Work out the finished part from the listing and answer in its coordinate system (mm). Coordinates: 2 decimals unless noted, no trailing zeros. Loops run counter-clockwise (first coordinate to the right, second up) from the corner with the lowest first, then second, coordinate; pieces in that order, holes last. Notation, with made-up numbers: (38.5, 25.5) -> (44.5, 25.5) arc R17 cw to (44.5, 41.5) -> close; hole circle Ø6 at (32.5, 43). An arc over 180 degrees is marked (long way). Use a Markdown table: item, result.
from build123d import *

# Parameters (mm, degrees)
CROQUIS1_W              = 250
CROQUIS1_H              = 150
SALIENTE_EXTRUIR1_DEPTH = 10
CORTAR_EXTRUIR1_REACH   = 12
CROQUIS2_R              = 12.5
CROQUIS2_R_2            = 15.5
CORTAR_EXTRUIR2_REACH   = 12
CROQUIS3_R              = 1.6


with BuildPart() as part:
    # Croquis1 → Saliente-Extruir1 (new body)
    with BuildSketch(Plane(origin=(0, 0, 0), x_dir=(1, 0, 0), z_dir=(0, 1, 0))):
        Rectangle(CROQUIS1_W, CROQUIS1_H)
    extrude(amount=SALIENTE_EXTRUIR1_DEPTH)

    # Croquis2 → Cortar-Extruir1 (cut, up to next)
    with BuildSketch(Plane(origin=(0, 10, 0), x_dir=(1, 0, 0), z_dir=(0, 1, 0)), mode=Mode.PRIVATE) as cortar_extruir1_sk1:
        with Locations((-73.102687588, -7.952940163)):
            Circle(CROQUIS2_R)
    cortar_extruir1_tool1 = extrude(cortar_extruir1_sk1.sketch, amount=-CORTAR_EXTRUIR1_REACH, mode=Mode.PRIVATE) & part.part
    add(cortar_extruir1_tool1.solids().sort_by_distance((-73.102688, 10, 7.95294))[0], mode=Mode.SUBTRACT)
    # Croquis2 → Cortar-Extruir1 (cut, up to next)
    with BuildSketch(Plane(origin=(0, 10, 0), x_dir=(1, 0, 0), z_dir=(0, 1, 0)), mode=Mode.PRIVATE) as cortar_extruir1_sk2:
        with Locations((-4.370803181, -26.878296525)):
            Circle(CROQUIS2_R_2)
    cortar_extruir1_tool2 = extrude(cortar_extruir1_sk2.sketch, amount=-CORTAR_EXTRUIR1_REACH, mode=Mode.PRIVATE) & part.part
    add(cortar_extruir1_tool2.solids().sort_by_distance((-4.370803, 10, 26.878297))[0], mode=Mode.SUBTRACT)
    # Croquis2 → Cortar-Extruir1 (cut, up to next)
    with BuildSketch(Plane(origin=(0, 10, 0), x_dir=(1, 0, 0), z_dir=(0, 1, 0)), mode=Mode.PRIVATE) as cortar_extruir1_sk3:
        with Locations((2.765040009, 12.93083036)):
            Circle(CROQUIS2_R_2)
    cortar_extruir1_tool3 = extrude(cortar_extruir1_sk3.sketch, amount=-CORTAR_EXTRUIR1_REACH, mode=Mode.PRIVATE) & part.part
    add(cortar_extruir1_tool3.solids().sort_by_distance((2.76504, 10, -12.93083))[0], mode=Mode.SUBTRACT)
    # Croquis2 → Cortar-Extruir1 (cut, up to next)
    with BuildSketch(Plane(origin=(0, 10, 0), x_dir=(1, 0, 0), z_dir=(0, 1, 0)), mode=Mode.PRIVATE) as cortar_extruir1_sk4:
        with Locations((39.781486463, 27.243051559)):
            Circle(CROQUIS2_R_2)
    cortar_extruir1_tool4 = extrude(cortar_extruir1_sk4.sketch, amount=-CORTAR_EXTRUIR1_REACH, mode=Mode.PRIVATE) & part.part
    add(cortar_extruir1_tool4.solids().sort_by_distance((39.781486, 10, -27.243052))[0], mode=Mode.SUBTRACT)
    # Croquis2 → Cortar-Extruir1 (cut, up to next)
    with BuildSketch(Plane(origin=(0, 10, 0), x_dir=(1, 0, 0), z_dir=(0, 1, 0)), mode=Mode.PRIVATE) as cortar_extruir1_sk5:
        with Locations((76.517860202, 27.243051559)):
            Circle(CROQUIS2_R_2)
    cortar_extruir1_tool5 = extrude(cortar_extruir1_sk5.sketch, amount=-CORTAR_EXTRUIR1_REACH, mode=Mode.PRIVATE) & part.part
    add(cortar_extruir1_tool5.solids().sort_by_distance((76.51786, 10, -27.243052))[0], mode=Mode.SUBTRACT)
    # Croquis2 → Cortar-Extruir1 (cut, up to next)
    with BuildSketch(Plane(origin=(0, 10, 0), x_dir=(1, 0, 0), z_dir=(0, 1, 0)), mode=Mode.PRIVATE) as cortar_extruir1_sk6:
        with Locations((68.851282971, -12.913044543)):
            Circle(CROQUIS2_R_2)
    cortar_extruir1_tool6 = extrude(cortar_extruir1_sk6.sketch, amount=-CORTAR_EXTRUIR1_REACH, mode=Mode.PRIVATE) & part.part
    add(cortar_extruir1_tool6.solids().sort_by_distance((68.851283, 10, 12.913045))[0], mode=Mode.SUBTRACT)
    # Croquis2 → Cortar-Extruir1 (cut, up to next)
    with BuildSketch(Plane(origin=(0, 10, 0), x_dir=(1, 0, 0), z_dir=(0, 1, 0)), mode=Mode.PRIVATE) as cortar_extruir1_sk7:
        with Locations((32.113542958, -12.913044543)):
            Circle(CROQUIS2_R_2)
    cortar_extruir1_tool7 = extrude(cortar_extruir1_sk7.sketch, amount=-CORTAR_EXTRUIR1_REACH, mode=Mode.PRIVATE) & part.part
    add(cortar_extruir1_tool7.solids().sort_by_distance((32.113543, 10, 12.913045))[0], mode=Mode.SUBTRACT)

    # Croquis3 → Cortar-Extruir2 (cut, up to next)
    with BuildSketch(Plane(origin=(0, 10, 0), x_dir=(1, 0, 0), z_dir=(0, 1, 0)), mode=Mode.PRIVATE) as cortar_extruir2_sk1:
        with Locations((-110, 59)):
            Circle(CROQUIS3_R)
    cortar_extruir2_tool1 = extrude(cortar_extruir2_sk1.sketch, amount=-CORTAR_EXTRUIR2_REACH, mode=Mode.PRIVATE) & part.part
    add(cortar_extruir2_tool1.solids().sort_by_distance((-110, 10, -59))[0], mode=Mode.SUBTRACT)
    # Croquis3 → Cortar-Extruir2 (cut, up to next)
    with BuildSketch(Plane(origin=(0, 10, 0), x_dir=(1, 0, 0), z_dir=(0, 1, 0)), mode=Mode.PRIVATE) as cortar_extruir2_sk2:
        with Locations((110, 59)):
            Circle(CROQUIS3_R)
    cortar_extruir2_tool2 = extrude(cortar_extruir2_sk2.sketch, amount=-CORTAR_EXTRUIR2_REACH, mode=Mode.PRIVATE) & part.part
    add(cortar_extruir2_tool2.solids().sort_by_distance((110, 10, -59))[0], mode=Mode.SUBTRACT)
    # Croquis3 → Cortar-Extruir2 (cut, up to next)
    with BuildSketch(Plane(origin=(0, 10, 0), x_dir=(1, 0, 0), z_dir=(0, 1, 0)), mode=Mode.PRIVATE) as cortar_extruir2_sk3:
        with Locations((110, -60)):
            Circle(CROQUIS3_R)
    cortar_extruir2_tool3 = extrude(cortar_extruir2_sk3.sketch, amount=-CORTAR_EXTRUIR2_REACH, mode=Mode.PRIVATE) & part.part
    add(cortar_extruir2_tool3.solids().sort_by_distance((110, 10, 60))[0], mode=Mode.SUBTRACT)
    # Croquis3 → Cortar-Extruir2 (cut, up to next)
    with BuildSketch(Plane(origin=(0, 10, 0), x_dir=(1, 0, 0), z_dir=(0, 1, 0)), mode=Mode.PRIVATE) as cortar_extruir2_sk4:
        with Locations((-110, -60)):
            Circle(CROQUIS3_R)
    cortar_extruir2_tool4 = extrude(cortar_extruir2_sk4.sketch, amount=-CORTAR_EXTRUIR2_REACH, mode=Mode.PRIVATE) & part.part
    add(cortar_extruir2_tool4.solids().sort_by_distance((-110, 10, 60))[0], mode=Mode.SUBTRACT)
    # Croquis3 → Cortar-Extruir2 (cut, up to next)
    with BuildSketch(Plane(origin=(0, 10, 0), x_dir=(1, 0, 0), z_dir=(0, 1, 0)), mode=Mode.PRIVATE) as cortar_extruir2_sk5:
        with Locations((-50.352687588, 34.767059837)):
            Circle(CROQUIS3_R)
    cortar_extruir2_tool5 = extrude(cortar_extruir2_sk5.sketch, amount=-CORTAR_EXTRUIR2_REACH, mode=Mode.PRIVATE) & part.part
    add(cortar_extruir2_tool5.solids().sort_by_distance((-50.352688, 10, -34.76706))[0], mode=Mode.SUBTRACT)
    # Croquis3 → Cortar-Extruir2 (cut, up to next)
    with BuildSketch(Plane(origin=(0, 10, 0), x_dir=(1, 0, 0), z_dir=(0, 1, 0)), mode=Mode.PRIVATE) as cortar_extruir2_sk6:
        with Locations((-50.352687588, -50.672940163)):
            Circle(CROQUIS3_R)
    cortar_extruir2_tool6 = extrude(cortar_extruir2_sk6.sketch, amount=-CORTAR_EXTRUIR2_REACH, mode=Mode.PRIVATE) & part.part
    add(cortar_extruir2_tool6.solids().sort_by_distance((-50.352688, 10, 50.67294))[0], mode=Mode.SUBTRACT)
    # Croquis3 → Cortar-Extruir2 (cut, up to next)
    with BuildSketch(Plane(origin=(0, 10, 0), x_dir=(1, 0, 0), z_dir=(0, 1, 0)), mode=Mode.PRIVATE) as cortar_extruir2_sk7:
        with Locations((-95.852687588, -50.672940163)):
            Circle(CROQUIS3_R)
    cortar_extruir2_tool7 = extrude(cortar_extruir2_sk7.sketch, amount=-CORTAR_EXTRUIR2_REACH, mode=Mode.PRIVATE) & part.part
    add(cortar_extruir2_tool7.solids().sort_by_distance((-95.852688, 10, 50.67294))[0], mode=Mode.SUBTRACT)
    # Croquis3 → Cortar-Extruir2 (cut, up to next)
    with BuildSketch(Plane(origin=(0, 10, 0), x_dir=(1, 0, 0), z_dir=(0, 1, 0)), mode=Mode.PRIVATE) as cortar_extruir2_sk8:
        with Locations((-95.852687588, 34.767059837)):
            Circle(CROQUIS3_R)
    cortar_extruir2_tool8 = extrude(cortar_extruir2_sk8.sketch, amount=-CORTAR_EXTRUIR2_REACH, mode=Mode.PRIVATE) & part.part
    add(cortar_extruir2_tool8.solids().sort_by_distance((-95.852688, 10, -34.76706))[0], mode=Mode.SUBTRACT)


solid = part.part
Q1. Determine the mould class of faces 1 (the flat face through (-30, 0, -1)), 2 (the flat face through (125, 5, 1)), 3 (the cylindrical face through (53.366, 5.07, 12.232)) for opening direction X: pulls with the +X half, pulls with the -X half, needs draft (parallel to the pull), parting line crosses it, or undercut.
Solved:
| item | result |
|---|---|
| face 1 | needs draft |
| face 2 | pulls with the +X half |
| face 3 | undercut |
Q2. Consider line 1 (X direction, y = 5.25, z = -59); line 2 (Z direction, x = 110, y = 7.25); line 3 (Z direction, x = -5, y = 7.25). Determine where each line is inside the solid, lowest interval first. Write a range as [from, to].
Solved:
| item | result |
|---|---|
| line 1 | [-125, -111.6], [-108.4, 108.4], [111.6, 125] |
| line 2 | [-75, -60.6], [-57.4, 58.4], [61.6, 75] |
| line 3 | [-75, -26.35], [0.48, 11.39], [42.37, 75] |
Q3. Section B-B on z = -8.5 is taken. Determine the outline of the cut face in (x, y), and give its area (3 significant figures).
Solved:
| item | result |
|---|---|
| outline | (-125, 0) -> (-12.09, 0) -> (-12.09, 10) -> (-125, 10) -> close; (17.62, 0) -> (125, 0) -> (125, 10) -> (17.62, 10) -> close |
| area | 2,200 mm² |
Q4. Section A-A on x = 65.5 is taken. Determine the outline of the cut face in (y, z).
Solved:
| item | result |
|---|---|
| outline | (0, -75) -> (10, -75) -> (10, -38.15) -> (0, -38.15) -> close; (0, -16.34) -> (10, -16.34) -> (10, -2.22) -> (0, -2.22) -> close; (0, 28.05) -> (10, 28.05) -> (10, 75) -> (0, 75) -> close |
Q5. Given pin 1 Ø3 at (x, z) = (110, -59) entering from -Y; pin 2 Ø4 at (x, z) = (-95.85, -34.77) entering from -Y, each flat-ended and moving along its own axis, determine where each tip first touches the part or whether it passes through.
Solved:
| item | result |
|---|---|
| pin 1 | through |
| pin 2 | y = 0 |
Q6. Section D-D on x = -6.5 is taken. Determine the outline of the cut face in (y, z), and give its area (3 significant figures).
Solved:
| item | result |
|---|---|
| outline | (0, -75) -> (10, -75) -> (10, -25.36) -> (0, -25.36) -> close; (0, -0.5) -> (10, -0.5) -> (10, 11.53) -> (0, 11.53) -> close; (0, 42.23) -> (10, 42.23) -> (10, 75) -> (0, 75) -> close |
| area | 944 mm² |
Q7. Section C-C on y = 8.5 is taken. State how many separate pieces and enclosed holes the cut face has, and give its area (3 significant figures).
Solved:
| item | result |
|---|---|
| separate pieces | 1 |
| enclosed holes | 15 |
| area | 32,400 mm² |
